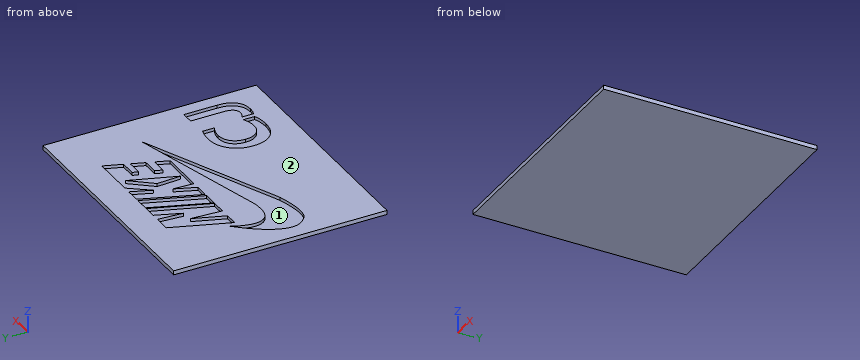
Autodesk Inventor part; units mm, degrees
ref_plane "YZ Plane" through (0, 0, 0) normal (1, 0, 0) x (0, 1, 0)
ref_plane "XZ Plane" through (0, 0, 0) normal (0, 1, 0) x (-1, 0, 0)
ref_plane "XY Plane" through (0, 0, 0) normal (0, 0, 1) x (1, 0, 0)
sketch "Boceto1" plane through (0, 0, 0) normal (0, 0, 1) x (1, 0, 0)
  line L0 (-250, -250) -> (250, -250)
  line L1 (250, -250) -> (250, 250)
  line L2 (250, 250) -> (-250, 250)
  line L3 (-250, 250) -> (-250, -250)
  line L4 (-250, -250) -> (250, 250) construction
  line L5 (250, -250) -> (-250, 250) construction
  point P0 (0, 0)
  dimension "d0" = 500
  dimension "d1" = 500
extrude "Extrusión1" add sketch "Boceto1" along normal blind 6
sketch "Boceto4" plane through (0, 0, 6) normal (0, 0, 1) x (1, 0, 0)
  line L0 (-122.9682, 69.533) -> (177.0318, 69.533) construction
  line L1 (177.0318, 69.533) -> (177.0318, -53.8632) construction
  line L2 (177.0318, -53.8632) -> (-122.9682, -53.8632) construction
  line L3 (-122.9682, -53.8632) -> (-122.9682, 69.533) construction
  line L4 (163.4789, 57.5416) -> (-40.9722, 2.948)
  spline S0 degree 4 poles (-40.9722, 2.948) (-59.3478, 1.0194) (-98.1126, -3.325) (-80.4924, 43.1707) (-72.4826, 57.5416) knots 0 0 0 0 0 1 1 1 1 1
  spline S1 degree 4 poles (-72.4826, 57.5416) (-101.0846, 27.8162) (-107.584, 11.7419) (-123.1576, -16.2785) (-102.1609, -32.5927) knots 0 0 0 0 0 1 1 1 1 1
  spline S2 degree 3 poles (-102.1609, -32.5927) (-92.0174, -46.5521) (-57.6708, -37.567) (-40.9722, -32.5927) knots 0 0 0 0 1 1 1 1
  line L5 (-40.9722, -32.5927) -> (163.4789, 57.5416)
  point P0 (0, 0)
  point P1 (-62.9545, 2.949)
  point P2 (-77.976, 12.1095)
  point P3 (-80.9081, 33.7265)
  point P4 (-98.8634, 24.932)
  point P5 (-109.4889, 2.9481)
  point P6 (-111.753, -15.9522)
  point P7 (-88.6041, -39.5543)
  point P8 (-62.956, -38.0886)
  dimension "d19" = 300
extrude "Extrusión4" cut sketch "Boceto4" against normal blind 4.5
sketch "Boceto6" plane through (0, 0, 6) normal (0, 0, 1) x (1, 0, 0)
  line L0 (82.2007, -20.2301) -> (276.8192, -20.2301) construction
  line L1 (276.8192, -20.2301) -> (276.8192, -107.8084) construction
  line L2 (276.8192, -107.8084) -> (82.2007, -107.8084) construction
  line L3 (82.2007, -107.8084) -> (82.2007, -20.2301) construction
  spline S0 degree 2 poles (148.6942, -98.7459) (139.9372, -102.9759) (125.8371, -102.9759) knots 0 0 0 1 1 1
  spline S1 degree 2 poles (125.8371, -102.9759) (107.4326, -102.9759) (86.3565, -81.3061) (86.3565, -63.2728) knots 0 0 0 1 2 2 2
  spline S2 degree 2 poles (86.3565, -63.2728) (86.3565, -44.052) (110.03, -20.2301) (128.9539, -20.2301) knots 0 0 0 1 2 2 2
  spline S3 degree 2 poles (128.9539, -20.2301) (140.6794, -20.2301) (148.6942, -23.1243) knots 0 0 0 1 1 1
  line L4 (148.6942, -23.1243) -> (148.6942, -40.4898)
  spline S4 degree 2 poles (148.6942, -40.4898) (140.6794, -35.7403) (130.4382, -35.7403) knots 0 0 0 1 1 1
  spline S5 degree 2 poles (130.4382, -35.7403) (119.158, -35.7403) (105.2805, -49.9147) (105.2805, -62.0112) knots 0 0 0 1 2 2 2
  spline S6 degree 2 poles (105.2805, -62.0112) (105.2805, -73.5882) (118.3417, -87.3915) (129.3992, -87.3915) knots 0 0 0 1 2 2 2
  spline S7 degree 2 poles (129.3992, -87.3915) (139.9372, -87.3915) (148.6942, -82.2709) knots 0 0 0 1 1 1
  line L5 (148.6942, -82.2709) -> (148.6942, -98.7459)
  spline S8 degree 2 poles (196.0411, -69.8034) (196.0411, -85.9073) (181.1246, -102.9759) (167.0244, -102.9759) knots 0 0 0 1 2 2 2
  spline S9 degree 2 poles (167.0244, -102.9759) (160.7165, -102.9759) (155.3732, -100.7496) knots 0 0 0 1 1 1
  line L6 (155.3732, -100.7496) -> (155.3732, -83.9036)
  spline S10 degree 2 poles (155.3732, -83.9036) (159.9744, -87.3915) (165.7629, -87.3915) knots 0 0 0 1 1 1
  spline S11 degree 2 poles (165.7629, -87.3915) (178.082, -87.3915) (178.082, -69.0613) knots 0 0 0 1 1 1
  line L7 (178.082, -69.0613) -> (178.082, -21.5659)
  line L8 (178.082, -21.5659) -> (196.0411, -21.5659)
  line L9 (196.0411, -21.5659) -> (196.0411, -69.8034)
  point P0 (0, 0)
extrude "Extrusión5" cut sketch "Boceto6" against normal blind 4.5
sketch "Boceto7" plane through (0, 0, 6) normal (0, 0, 1) x (1, 0, 0)
  line L0 (-96.8701, 190.9254) -> (156.7066, 190.9254) construction
  line L1 (156.7066, 190.9254) -> (156.7066, -16.508) construction
  line L2 (156.7066, -16.508) -> (-96.8701, -16.508) construction
  line L3 (-96.8701, -16.508) -> (-96.8701, 190.9254) construction
  line L4 (-67.4617, 47.7989) -> (-48.6104, 47.7989)
  line L5 (-48.6104, 47.7989) -> (-31.9884, 92.9574)
  line L6 (-31.9884, 92.9574) -> (-34.8888, 47.7989)
  line L7 (-34.8888, 47.7989) -> (-13.9857, 47.7989)
  line L8 (-13.9857, 47.7989) -> (16.5477, 130.7517)
  line L9 (16.5477, 130.7517) -> (-2.1497, 130.7517)
  line L10 (-13.3744, 130.7517) -> (-36.9283, 130.7517)
  line L11 (-36.9283, 130.7517) -> (-67.4617, 47.7989)
  line L12 (7.7072, 47.7989) -> (-12.5423, 47.7989)
  line L13 (-12.5423, 47.7989) -> (18.6965, 130.7517)
  line L14 (18.6965, 130.7517) -> (38.946, 130.7517)
  line L15 (38.946, 130.7517) -> (7.7072, 47.7989)
  line L16 (-13.3744, 130.7517) -> (-16.165, 94.0996)
  line L17 (-2.1497, 130.7517) -> (-16.165, 94.0996)
  line L18 (42.7507, 130.7517) -> (63.3753, 130.7517)
  line L19 (63.3753, 130.7517) -> (51.8446, 101.3389)
  line L20 (51.8446, 101.3389) -> (73.7311, 130.7517)
  line L21 (73.7311, 130.7517) -> (135.5179, 130.7517)
  line L22 (135.5179, 130.7517) -> (125.7617, 104.2462)
  line L23 (125.7617, 104.2462) -> (103.1886, 104.2462)
  line L24 (103.1886, 104.2462) -> (100.257, 96.2815)
  line L25 (100.257, 96.2815) -> (122.8301, 96.2815)
  line L26 (122.8301, 96.2815) -> (115.7727, 77.108)
  line L27 (115.7727, 77.108) -> (93.1995, 77.108)
  line L28 (93.1995, 77.108) -> (89.4446, 66.9066)
  line L29 (89.4446, 66.9066) -> (112.0177, 66.9066)
  line L30 (112.0177, 66.9066) -> (104.9845, 47.7989)
  line L31 (104.9845, 47.7989) -> (41.2278, 47.7989)
  line L32 (41.2278, 47.7989) -> (42.6118, 77.7874)
  line L33 (42.6118, 77.7874) -> (30.8554, 47.7989)
  line L34 (11.0305, 47.7989) -> (42.7507, 130.7517)
  line L35 (30.8554, 47.7989) -> (11.0305, 47.7989)
  line L36 (89.4446, 121.013) -> (65.5232, 54.1821)
  line L37 (65.5232, 54.1821) -> (63.9179, 89.2753)
  line L38 (63.9179, 89.2753) -> (89.4446, 121.013)
  point P0 (0, 0)
extrude "Extrusión6" cut sketch "Boceto7" against normal blind 4.5
sketch "Boceto8" plane through (0, 0, 6) normal (0, 0, 1) x (1, 0, 0)
  line L0 (-134.2632, 172.8911) -> (215.2572, 172.8911)
  line L1 (215.2572, 172.8911) -> (215.2572, -137.3783)
  line L2 (215.2572, -137.3783) -> (-134.2632, -137.3783)
  line L3 (-134.2632, -137.3783) -> (-134.2632, 172.8911)
  line L4 (250, 250) -> (-250, 250)
  line L5 (250, -250) -> (250, 250)
  line L6 (-250, 250) -> (250, 250)
  line L7 (250, 250) -> (250, -250)
  line L8 (250, -250) -> (-250, -250)
  line L9 (-250, -250) -> (-250, 250)
  point P0 (0, 0)
extrude "Extrusión7" cut sketch "Boceto8" against normal blind 133.25
equation "\"d1\" = d0"
properties part number "Silueta_nike_nombres"
Geometry check sheet. Reference: the model listing, model coordinates, mm. Face numbers are marked on the shaded views. Round coordinates to 2 decimals unless told otherwise and drop trailing zeros. Loops run counter-clockwise (first coordinate to the right, second up) from the corner with the lowest first, then second, coordinate; pieces in that order, holes last. Notation, with made-up numbers: (81, -20) - (88, -20) arc R27 ccw to (88, 12) - close; hole circle Ø4 at (33.25, 51.5). An arc over 180 degrees is marked (long way). Answer as CSV lines item,"result".
(1) Depth check by flat-ended pin: pin 1 Ø10 at (x, y) = (105, 110.5) entering from +Z. Enter the tip coordinate at first touch or a pass-through.
Output values:
pin 1,"stops at z = 1.5"
(2) Cross-section at A-A, the plane z = 4.25. Give the number of separate pieces and of enclosed holes in the cut face, and give its area (3 significant figures).
Output values:
separate pieces,"2"
enclosed holes,"6"
area,"84,800 mm²"
(3) Cross-section at C-C, the plane y = 110.5. Enter the section's corners in (x, z).
Output values:
outline,"(-134.26, 0) - (215.26, 0) - (215.26, 6) - (128.06, 6) - (128.06, 1.5) - (85.68, 1.5) - (85.68, 6) - (80.99, 6) - (80.99, 1.5) - (58.66, 1.5) - (58.66, 6) - (55.44, 6) - (55.44, 1.5) - (35.01, 1.5) - (35.01, 6) - (31.32, 6) - (31.32, 1.5) - (11.07, 1.5) - (11.07, 6) - (9.09, 6) - (9.09, 1.5) - (-9.89, 1.5) - (-9.89, 6) - (-14.92, 6) - (-14.92, 1.5) - (-44.38, 1.5) - (-44.38, 6) - (-134.26, 6) - close"
(4) Material ranges on line 1 along Y through (x, z) = (146, 5); line 2 along X through (y, z) = (87.5, 5.75); line 3 along X through (y, z) = (-98, 4.25), recorded low to high.
Output values:
line 1,"y = -137.38 to -99.9, -83.7 to -39.06, -22.26 to 49.84, 52.87 to 172.89"
line 2,"x = -134.26 to -52.85, -34 to -32.34, 0.63 to 2.41, 22.66 to 26.21, 64 to 77.45, 119.6 to 215.26"
line 3,"x = -134.26 to 104.51, 148.69 to 155.37, 184.68 to 215.26"
(5) Cross-section at B-B, the plane x = 47.5. Enter the section's corners in (y, z).
Output values:
outline,"(-137.38, 0) - (172.89, 0) - (172.89, 6) - (130.75, 6) - (130.75, 1.5) - (47.8, 1.5) - (47.8, 6) - (26.57, 6) - (26.57, 1.5) - (6.41, 1.5) - (6.41, 6) - (-137.38, 6) - close"
(6) Release check for a two-part mould opening along X. For the marked faces 1 and 2 record: released by +X, released by -X, zero draft, split by the parting line, or undercut.
Output values:
face 1,"undercut"
face 2,"zero draft"
